from build123d import *

# Parameters (mm, degrees)
SKETCH1_R             = 1.75
BOSS_EXTRUDE1_DEPTH   = 5
BOSS_EXTRUDE1_2_DEPTH = 5
SKETCH1_2_R           = 1.75
BOSS_EXTRUDE2_DEPTH   = 5
BOSS_EXTRUDE3_DEPTH   = 35


with BuildPart() as part:
    # Sketch1 → Boss-Extrude1 (new body)
    with BuildSketch(Plane.XY):
        Polygon((-3, 3), (5.1, 3), (5.1, -32), (-3, -32), (-3, -26), align=None)
        Circle(SKETCH1_R, mode=Mode.SUBTRACT)
        with Locations(Location((0, -29, 0), (0, 0, 180))):
            Circle(SKETCH1_R, mode=Mode.SUBTRACT)
    extrude(amount=BOSS_EXTRUDE1_DEPTH)



with BuildPart() as body_2:
    # Sketch1 → Boss-Extrude1 2 (new body)
    with BuildSketch(Plane.XY):
        Polygon((50.27, 3), (42.17, 3), (42.17, -32), (50.27, -32), (50.27, -26), align=None)
        with Locations((47.27, 0)):
            Circle(SKETCH1_R, mode=Mode.SUBTRACT)
        with Locations(Location((47.27, -29, 0), (0, 0, 180))):
            Circle(SKETCH1_R, mode=Mode.SUBTRACT)
    extrude(amount=BOSS_EXTRUDE1_2_DEPTH)


with BuildPart() as part_1:
    add(part.part)

    add(body_2.part)  # Boss-Extrude2 merges body 2
    # Sketch1<2> → Boss-Extrude2 (add)
    # profile 1 of 2: a face of its own
    with BuildSketch(Plane.XY):
        Polygon((-3, 3), (5.1, 3), (5.1, -32), (-3, -32), (-3, -26), align=None)
        Circle(SKETCH1_2_R, mode=Mode.SUBTRACT)
        with Locations(Location((0, -29, 0), (0, 0, 180))):
            Circle(SKETCH1_2_R, mode=Mode.SUBTRACT)
    # profile 2 of 2: a face of its own
    with BuildSketch(Plane.XY):
        Polygon((50.27, 3), (42.17, 3), (42.17, -32), (50.27, -32), (50.27, -26), align=None)
        with Locations((47.27, 0)):
            Circle(SKETCH1_2_R, mode=Mode.SUBTRACT)
        with Locations(Location((47.27, -29, 0), (0, 0, 180))):
            Circle(SKETCH1_2_R, mode=Mode.SUBTRACT)
    extrude(amount=BOSS_EXTRUDE2_DEPTH)

    # Sketch2 → Boss-Extrude3 (add)
    with BuildSketch(Plane(origin=(0, 3, 0), x_dir=(1, 0, 0), z_dir=(0, 1, 0))):
        with BuildLine():
            Line((42.17, 0), (44.305, 0))
            ThreePointArc((44.305, 0), (23.635, -20.67), (2.965, 0))
            Line((2.965, 0), (5.1, 0))
            ThreePointArc((5.1, 0), (23.635, -18.535), (42.17, 0))
        make_face()
    extrude(amount=-BOSS_EXTRUDE3_DEPTH)


solid = part_1.part
For this review, take the finished solid that the model builds, in its own axes (mm). A direction names the side the tool comes from. Give positions to 0.01 mm unless a question says otherwise; leave off trailing zeros. Order: outer loops, then holes, each group sorted by start corner. A loop starts at its lowest first (then second) coordinate and runs counter-clockwise, first axis right, second up. Notation, with made-up numbers: (-27, 68) -> (14, 68) arc R18 cw to (14, 79) -> close; hole circle Ø7 at (27.25, -8). An arc over 180 degrees is marked (long way). Write item = value, one per line.
1) We need section B-B, the plane y = 0. Give the boundary of the cut face in (x, z) (3 decimals).
Findings:
outline = (-3, 0) -> (-1.75, 0) -> (-1.75, 5) -> (-3, 5) -> close; (1.75, 0) -> (5.1, 0) arc R18.535 cw to (42.17, 0) -> (45.52, 0) -> (45.52, 5) -> (43.691, 5) arc R20.67 ccw to (3.579, 5) -> (1.75, 5) -> close; (49.02, 0) -> (50.27, 0) -> (50.27, 5) -> (49.02, 5) -> close
2) We need section A-A, the plane x = 47.27. Give the boundary of the cut face in (y, z), and give its area (3 significant figures).
Findings:
outline = (-32, 0) -> (-30.75, 0) -> (-30.75, 5) -> (-32, 5) -> close; (-27.25, 0) -> (-1.75, 0) -> (-1.75, 5) -> (-27.25, 5) -> close; (1.75, 0) -> (3, 0) -> (3, 5) -> (1.75, 5) -> close
area = 140 mm^2
3) We need section D-D, the plane x = 34.5. Give the boundary of the cut face in (y, z), and give its area (3 significant figures).
Findings:
outline = (-32, 15.02) -> (3, 15.02) -> (3, 17.58) -> (-32, 17.58) -> close
area = 89.9 mm^2
4) Draft analysis for pull direction Y (two halves, no side actions). For faces 1 (the face through (24, 3, 19)), 2 (the face through (48.887, -0.67, 2.465)), 3 (the face through (24.019, -14.255, 20.666)), 4 (the face through (45.653, -28.33, 2.465)), state which applies: pulls with the +Y half, pulls with the -Y half, needs draft (parallel to the pull), parting line crosses it, or undercut.
Findings:
face_1 = pulls with the +Y half
face_2 = undercut
face_3 = needs draft
face_4 = undercut
5) For faces 5 (the face through (1.617, -0.67, 2.465)), 6 (the face through (47, -14, 5)), 7 (the face through (0, -14, 5)), list the 3-axis set-ups (+Z, -Z, +X, -X, +Y, -Y) from which the entire face can be reached by the end or side of a thin tool; tool diameter is ignored.
Findings:
face_5 = +Z, -Z
face_6 = +Z, +X, +Y, -Y
face_7 = +Z, -X, +Y, -Y
6) To check wall thickness, follow L1, parallel to Y at x = 47.27, z = 1.5; L2, parallel to Z at x = 48, y = -4.5; L3, parallel to X at y = -13.5, z = 12.75. State the ranges of each line that lie inside material, in increasing order. Write a range as from..to.
Findings:
L1 = -32..-30.75, -27.25..-1.75, 1.75..3
L2 = 0..5
L3 = 7.37..10.18, 37.09..39.9
7) We need section C-C, the plane y = -6.5. Give the boundary of the cut face in (x, z) (3 decimals), and give its area (3 significant figures).
Findings:
outline = (-3, 0) -> (5.1, 0) arc R18.535 cw to (42.17, 0) -> (50.27, 0) -> (50.27, 5) -> (43.691, 5) arc R20.67 ccw to (3.579, 5) -> (-3, 5) -> close
area = 193 mm^2
8) Insertion check: pin 1 (2 mm diameter, centred on x = 30.5, y = -27.5, fed in from +Z); pin 2 (5.5 mm diameter, centred on x = 0, y = -8, fed in from +Z); pin 3 (5 mm diameter, centred on x = 21.5, y = -24.5, fed in from -Z). Each pin has a flat end and moves straight along its axis. Give the tip position at first contact, or say it passes through.
Findings:
pin_1 = 19.82
pin_2 = 5
pin_3 = 17.95
